Design review of the part built by this model. Coordinates are the model's own, in mm. A direction names the side the tool comes from. Round coordinates to 2 decimals unless told otherwise and drop trailing zeros. Loops run counter-clockwise (first coordinate to the right, second up) from the corner with the lowest first, then second, coordinate; pieces in that order, holes last. Notation, with made-up numbers: (49, 6) -> (91, 6) arc R11 ccw to (91, 17) -> close; hole circle Ø10 at (22, 10). An arc over 180 degrees is marked (long way). Answer as CSV lines item,"result". Start each with the question number.
```python
from build123d import *

# Parameters (mm, degrees)
F0_W     = 152.4
F0_H     = 76.2
F1_DEPTH = 12.7
F2_R     = 6.35
F3_DEPTH = 12.701
F4_DEPTH = 12.701
F5_DEPTH = 12.701
F6_DEPTH = 12.701
F7_W     = 25.4
F7_H     = 50.8
F9_W     = 10.16
F9_H     = 25.4
F11_R    = 2.54
F12_SIZE = 2.54


with BuildPart() as f1:
    # F0 (on Top) → F1 (new body)
    with BuildSketch(Plane.XY):
        Rectangle(F0_W, F0_H)
    extrude(amount=F1_DEPTH)

    # F2 (on face) → F3 (cut, through all)
    with BuildSketch(Plane.XY.offset(12.7)):
        with Locations((57.15, -25.4)):
            Circle(F2_R)
    extrude(amount=-F3_DEPTH, mode=Mode.SUBTRACT)

    # F2 (on face) → F4 (cut, through all)
    with BuildSketch(Plane.XY.offset(12.7)):
        with Locations((63.5, 25.4)):
            Circle(F2_R)
    extrude(amount=-F4_DEPTH, mode=Mode.SUBTRACT)

    # F2 (on face) → F5 (cut, through all)
    with BuildSketch(Plane.XY.offset(12.7)):
        with Locations((-63.5, -25.4)):
            Circle(F2_R)
    extrude(amount=-F5_DEPTH, mode=Mode.SUBTRACT)

    # F2 (on face) → F6 (cut, through all)
    with BuildSketch(Plane.XY.offset(12.7)):
        with Locations((-63.5, 25.4)):
            Circle(F2_R)
    extrude(amount=-F6_DEPTH, mode=Mode.SUBTRACT)

    # F7 (on Front) → F8 (revolve)
    with BuildSketch(Plane.XZ):
        with Locations((12.7, 38.1)):
            Rectangle(F7_W, F7_H)
    revolve(axis=Axis((0, 0, 38.1), (0, 0, -1)))

    # F9 (on Front) → F10 (revolve, cut)
    with BuildSketch(Plane.XZ):
        with Locations((-25.2770464867, 38.1)):
            Rectangle(F9_W, F9_H)
    revolve(axis=Axis((0, 0, 38.1), (0, 0, -1)), mode=Mode.SUBTRACT)

    # F11
    f11_edges = [f1.edges().sort_by_distance(p)[0] for p in [
        (-25.4, 0, 12.7),
        (-25.4, 0, 25.4),
        (-25.4, 0, 63.5),
    ]]
    fillet(f11_edges, radius=F11_R)

    # F12
    f12_edges = [f1.edges().sort_by_distance(p)[0] for p in [
        (0, -38.1, 12.7),
        (-76.2, 0, 12.7),
        (0, 38.1, 12.7),
        (76.2, 0, 12.7),
    ]]
    chamfer(f12_edges, length=F12_SIZE)


solid = f1.part
```
Q1. For pin 1 Ø1 at (y, z) = (21.5, 55) entering from +X; pin 2 Ø8 at (x, z) = (18, 39.5) entering from +Y; pin 3 Ø3 at (x, y) = (45, -30.5) entering from +Z, all flat-tipped, find the tip position at first contact; note any pin that passes through.
Q2. Add section B-B, the plane y = 0. Give the boundary of the cut face in (x, z), and give its area (3 significant figures).
Q3. Add section C-C, the plane z = 54. Give the boundary of the cut face in (x, y).
Q4. Machinability: for faces 5 (the flat face through (-8, -19, 25.4)), 6 (the cylindrical face through (-5.506, 24.796, 55.951)), 7 (the flat face through (-1, 1, 0)), which of the approach directions +Z, -Z, +X, -X, +Y, -Y give a long, thin tool a straight path to every point of the face, cutting with its end or side? Answer none if there is none.
Q5. Mouldability with a two-part tool opening along Y and no side actions: class faces 1 (the flat face through (0, 0, 63.5)), 2 (the flat face through (-1, -38.1, 5)), 3 (the cylindrical face through (-5.506, 24.796, 19.103)), 4 (the cylindrical face through (62.12, 19.2, 6.44)) as pulls with the +Y half, pulls with the -Y half, needs draft (parallel to the pull), parting line crosses it, or undercut.
Q6. Add section A-A, the plane x = 0. Give the boundary of the cut face in (y, z).
Q7. To check wall thickness, follow probe 1 along X at (y, z) = (25, 6); probe 2 along Y at (x, z) = (-63, 8); probe 3 along X at (y, z) = (-25, 5). State the ranges of each line that lie inside material, in increasing order. Write a range as from..to.
Q8. Add section D-D, the plane z = 31. Give the boundary of the cut face in (x, y).
Worked answers:
1,pin 1,"stops at x = 14.29"
1,pin 2,"stops at y = 14.56"
1,pin 3,"stops at z = 12.7"
2,outline,"(-76.2, 0) -> (76.2, 0) -> (76.2, 10.16) -> (73.66, 12.7) -> (27.94, 12.7) arc R2.54 cw to (25.4, 15.24) -> (25.4, 22.86) arc R2.54 ccw to (22.86, 25.4) -> (20.2, 25.4) -> (20.2, 50.8) -> (25.4, 50.8) -> (25.4, 60.96) arc R2.54 ccw to (22.86, 63.5) -> (-22.86, 63.5) arc R2.54 ccw to (-25.4, 60.96) -> (-25.4, 50.8) -> (-20.2, 50.8) -> (-20.2, 25.4) -> (-22.86, 25.4) arc R2.54 ccw to (-25.4, 22.86) -> (-25.4, 15.24) arc R2.54 cw to (-27.94, 12.7) -> (-73.66, 12.7) -> (-76.2, 10.16) -> close"
2,area,"4,240 mm^2"
3,outline,"circle Ø50.8 at (0, 0)"
4,face 5,"none"
4,face 6,"+Z"
4,face 7,"-Z, +X, -X, +Y, -Y"
5,face 1,"needs draft"
5,face 2,"pulls with the -Y half"
5,face 3,"parting line crosses it"
5,face 4,"undercut"
6,outline,"(-38.1, 0) -> (38.1, 0) -> (38.1, 10.16) -> (35.56, 12.7) -> (27.94, 12.7) arc R2.54 cw to (25.4, 15.24) -> (25.4, 22.86) arc R2.54 ccw to (22.86, 25.4) -> (20.2, 25.4) -> (20.2, 50.8) -> (25.4, 50.8) -> (25.4, 60.96) arc R2.54 ccw to (22.86, 63.5) -> (-22.86, 63.5) arc R2.54 ccw to (-25.4, 60.96) -> (-25.4, 50.8) -> (-20.2, 50.8) -> (-20.2, 25.4) -> (-22.86, 25.4) arc R2.54 ccw to (-25.4, 22.86) -> (-25.4, 15.24) arc R2.54 cw to (-27.94, 12.7) -> (-35.56, 12.7) -> (-38.1, 10.16) -> close"
7,probe 1,"x = -76.2..-69.84, -57.16..57.16, 69.84..76.2"
7,probe 2,"y = -38.1..-31.73, -19.07..19.07, 31.73..38.1"
7,probe 3,"x = -76.2..-69.84, -57.16..50.81, 63.49..76.2"
8,outline,"circle Ø40.39 at (0, 0)"
